from build123d import *

# Parameters (mm, degrees)
SKETCH1_R           = 2.5
BOSS_EXTRUDE1_DEPTH = 6


with BuildPart() as part:
    # Sketch1 → Boss-Extrude1 (new body)
    with BuildSketch(Plane.XY):
        Polygon((257.640643246, 162.769630368), (277.640643246, 142.769630368), (277.640643246, 82.769630368), (252.640643246, 82.769630368), (232.640643246, 102.769630368), (-367.359356754, 102.769630368), (-367.359356754, 162.769630368), align=None)
        with Locations((267.640643246, 105.769630368)):
            Circle(SKETCH1_R, mode=Mode.SUBTRACT)
        with Locations((267.640643246, 92.769630368)):
            Circle(SKETCH1_R, mode=Mode.SUBTRACT)
    extrude(amount=BOSS_EXTRUDE1_DEPTH)


solid = part.part
Design review of the part built by this model. Coordinates are the model's own, in mm. Round coordinates to 2 decimals unless told otherwise and drop trailing zeros. Write each loop counter-clockwise with the first axis right and the second up, starting at its lowest first coordinate (ties: lowest second). Pieces come first, ordered by that corner, then holes. Notation, with made-up numbers: (-12, -34) - (33, -34) arc R36 ccw to (33, 2) - close; hole circle Ø9 at (59, 86.5). An arc over 180 degrees is marked (long way). Use a Markdown table: item, result. Add a question column.
1. We need section A-A (z = 2.3). State the section outline as (x, y) points.
2. Wall thickness on probe 1 along X at (y, z) = (105, 2.45); probe 2 along Y at (x, z) = (118.5, 1.15); probe 3 along X at (y, z) = (103.5, 4.65): over which ranges is each line inside the solid? List them lowest first.
3. We need section B-B (x = -231.5). State the section outline as (y, z) points, then the cut area to 3 significant figures.
Output:
| question | item | result |
|---|---|---|
| 1 | outline | (-367.36, 102.77) - (232.64, 102.77) - (252.64, 82.77) - (277.64, 82.77) - (277.64, 142.77) - (257.64, 162.77) - (-367.36, 162.77) - close; hole circle Ø5 at (267.64, 92.77); hole circle Ø5 at (267.64, 105.77) |
| 2 | probe 1 | x = -367.36 to 265.26, 270.02 to 277.64 |
| 2 | probe 2 | y = 102.77 to 162.77 |
| 2 | probe 3 | x = -367.36 to 266.59, 268.69 to 277.64 |
| 3 | outline | (102.77, 0) - (162.77, 0) - (162.77, 6) - (102.77, 6) - close |
| 3 | area | 360 mm2 |
